```python
from build123d import *

# Parameters (mm, degrees)
SKETCH1_R                       = 24.1
BOSS_EXTRUDE1_DEPTH             = 10
TAP_DRILL_FOR_M5X0_8_TAP1_D     = 4.2
TAP_DRILL_FOR_M4X0_7_TAP1_D     = 3.3
SKETCH9_W                       = 55
SKETCH9_H                       = 45
BOSS_EXTRUDE2_DEPTH             = 4
TAP_DRILL_FOR_M5X0_8_TAP2_D     = 4.2
TAP_DRILL_FOR_M5X0_8_TAP2_DEPTH = 10
TAP_DRILL_FOR_M5X0_8_TAP2_TIP   = 1.2618073
FILLET1_R                       = 50


with BuildPart() as part:
    # Sketch1 → Boss-Extrude1 (new body)
    with BuildSketch(Plane.XY):
        with BuildLine():
            Line((-27.5, -28.354893758), (-27.5, -45.5))
            Line((-27.5, -45.5), (27.5, -45.5))
            Line((27.5, -45.5), (27.5, -28.354893758))
            ThreePointArc((27.5, -28.354893758), (0, 39.5), (-27.5, -28.354893758))
        make_face()
        Circle(SKETCH1_R, mode=Mode.SUBTRACT)
    extrude(amount=BOSS_EXTRUDE1_DEPTH)

    # Tap Drill for M5x0.8 Tap1 (through all)
    with Locations(Plane(origin=(23.573172318, 23.573172318, 0), x_dir=(-1, 0, 0), z_dir=(0, 0, -1))):
        with Locations((0, 0), (47.146344636, 0), (47.146344636, -47.146344636), (0, -47.146344636)):
            Hole(TAP_DRILL_FOR_M5X0_8_TAP1_D / 2)

    # Tap Drill for M4x0.7 Tap1 (through all)
    with Locations(Plane(origin=(-30.743901834, -17.75, 10), x_dir=(1, 0, 0), z_dir=(0, 0, 1))):
        with Locations((0, 0), (0, 35.5), (61.487803668, 35.5), (61.487803668, 0)):
            Hole(TAP_DRILL_FOR_M4X0_7_TAP1_D / 2)

    # Sketch9 → Boss-Extrude2 (add)
    with BuildSketch(Plane.XZ.offset(45.5)):
        with Locations((0, 22.5)):
            Rectangle(SKETCH9_W, SKETCH9_H)
    extrude(amount=BOSS_EXTRUDE2_DEPTH)

    # Tap Drill for M5x0.8 Tap2
    with Locations(Plane(origin=(-22.5, -49.5, 40.15274255), x_dir=(0, 0, -1), z_dir=(0, -1, 0))):
        with Locations((0, 0), (0, 45), (35, 45), (35, 0)):
            Hole(TAP_DRILL_FOR_M5X0_8_TAP2_D / 2, depth=TAP_DRILL_FOR_M5X0_8_TAP2_DEPTH)
            with Locations((0, 0, -(TAP_DRILL_FOR_M5X0_8_TAP2_DEPTH + TAP_DRILL_FOR_M5X0_8_TAP2_TIP / 2))):  # 118° drill point
                Cone(0, TAP_DRILL_FOR_M5X0_8_TAP2_D / 2, TAP_DRILL_FOR_M5X0_8_TAP2_TIP, mode=Mode.SUBTRACT)

    # Fillet1
    fillet1_edges = [part.edges().sort_by_distance(p)[0] for p in [
        (-27.5, -28.354893758, 5),
        (27.5, -28.354893758, 5),
    ]]
    fillet(fillet1_edges, radius=FILLET1_R)


solid = part.part
```
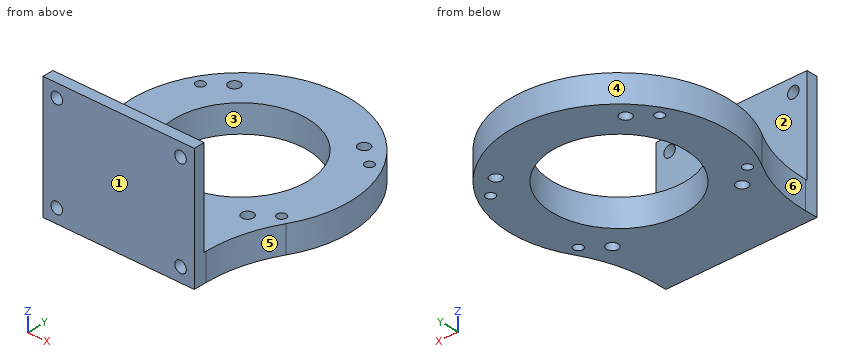
For this review, take the finished solid that the model builds, in its own axes (mm). Face numbers are marked on the shaded views. A direction names the side the tool comes from. Coordinates: 2 decimals unless noted, no trailing zeros. Loops run counter-clockwise (first coordinate to the right, second up) from the corner with the lowest first, then second, coordinate; pieces in that order, holes last. Notation, with made-up numbers: (-36, 38.25) - (11, 38.25) arc R20 ccw to (11, 44.25) - close; hole circle Ø5 at (-3.5, -31.5). An arc over 180 degrees is marked (long way). Use one line per item in the form item = value. Start each with the question number.
1) To check wall thickness, follow probe 1 along Z at (x, y) = (22.5, -42.75); probe 2 along Y at (x, z) = (1.5, 15.5); probe 3 along Y at (x, z) = (14.5, 5). State the ranges of each line that lie inside material, in increasing order. Write a range as from..to.
2) Take a section at B-B (x = 6). State the section outline as (y, z) points, plus the area to 3 significant figures.
3) Take a section at C-C (y = 17.75). State the section outline as (x, z) points.
4) For the marked faces 1 and 2, list the 3-axis set-ups (+Z, -Z, +X, -X, +Y, -Y) from which the entire face can be reached by the end or side of a thin tool; tool diameter is ignored.
5) Take a section at A-A (y = 0). State the section outline as (x, z) points.
6) Take a section at D-D (z = 12). State the section outline as (x, y) points, plus the area to 3 significant figures.
7) Draft analysis for pull direction X (two halves, no side actions). For the marked faces 3, 4, 5 and 6, state which applies: released by +X, released by -X, zero draft, split by the parting line, or undercut.
8) For pin 1 (1 mm diameter, centred on x = -24, y = -12.5, fed in from -Z); pin 2 (2 mm diameter, centred on y = -21, z = 9.5, fed in from -X); pin 3 (1.4 mm diameter, centred on y = -47, z = 32.5, fed in from +X), all flat-tipped, find the tip position at first contact; note any pin that passes through.
From the geometry:
q1.probe_1 = 0..3.05, 7.25..10
q1.probe_2 = -49.5..-45.5
q1.probe_3 = -49.5..-19.25, 19.25..36.74
q2.outline = (-49.5, 0) - (-23.34, 0) - (-23.34, 10) - (-45.5, 10) - (-45.5, 45) - (-49.5, 45) - close; (23.34, 0) - (39.04, 0) - (39.04, 10) - (23.34, 10) - close
q2.area = 559 mm2
q3.outline = (-35.29, 0) - (-32.39, 0) - (-32.39, 10) - (-35.29, 10) - close; (-29.09, 0) - (-16.3, 0) - (-16.3, 10) - (-29.09, 10) - close; (16.3, 0) - (29.09, 0) - (29.09, 10) - (16.3, 10) - close; (32.39, 0) - (35.29, 0) - (35.29, 10) - (32.39, 10) - close
q4.face_1 = +Z, -Z, +X, -X, -Y
q4.face_2 = +Z, +X, -X, +Y
q5.outline = (-39.5, 0) - (-24.1, 0) - (-24.1, 10) - (-39.5, 10) - close; (24.1, 0) - (39.5, 0) - (39.5, 10) - (24.1, 10) - close
q6.outline = (-27.5, -49.5) - (27.5, -49.5) - (27.5, -45.5) - (-27.5, -45.5) - close
q6.area = 220 mm2
q7.face_3 = undercut
q7.face_4 = split by the parting line
q7.face_5 = released by +X
q7.face_6 = released by -X
q8.pin_1 = 0
q8.pin_2 = -34.06
q8.pin_3 = 27.5
